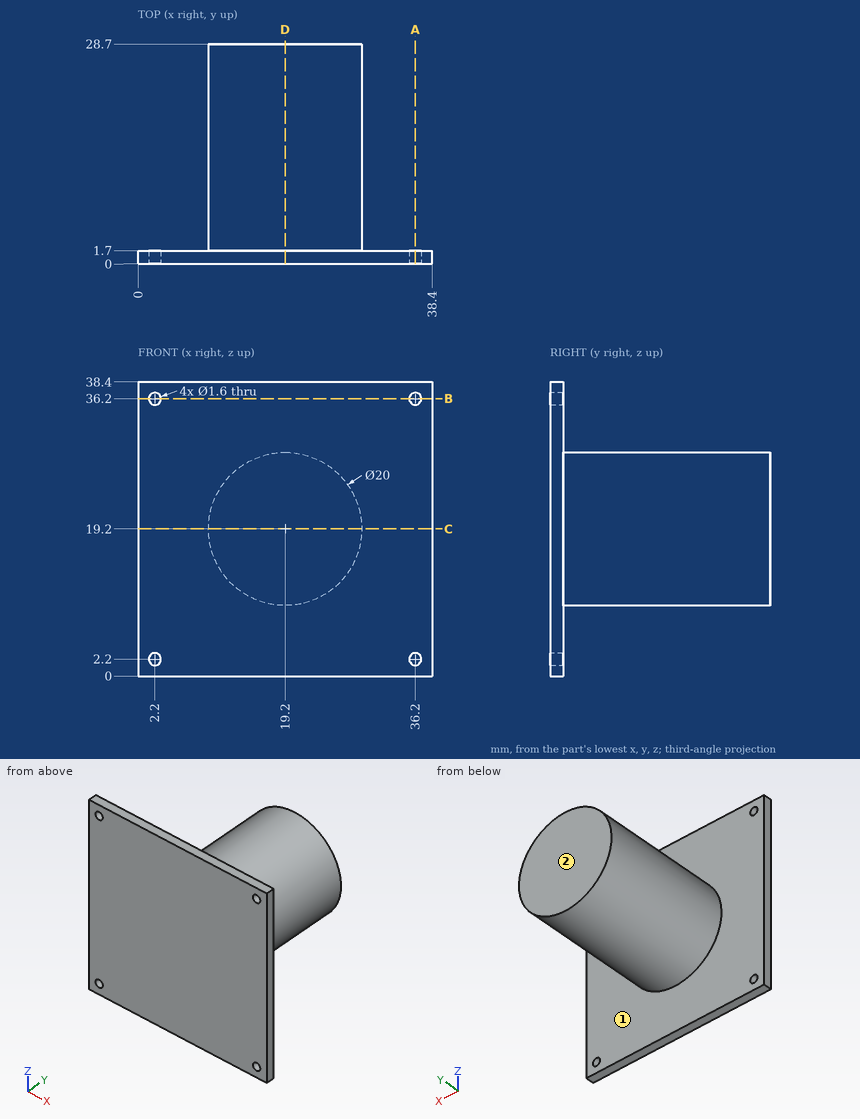
Geometry: see drawing. Coordinates: mm, zero at the bounding-box minimum. A direction names the side the tool comes from. Round coordinates to 2 decimals unless told otherwise and drop trailing zeros. Write each loop counter-clockwise with the first axis right and the second up, starting at its lowest first coordinate (ties: lowest second). Pieces come first, ordered by that corner, then holes.
Item 1: Material intervals for L1, parallel to X at y = 0.55, z = 2.2; L2, parallel to Y at x = 27, z = 4.5, sorted ascending.
Item 2: Section query A-A (x = 36.2). Return loops of the section in (y, z).
Item 3: Pin query (flat end, axial travel): P1, Ø1, axis at x = 24.5, z = 31, coming from the +Y side; P2, Ø1, axis at y = 7.5, z = 8.5, coming from the -X side. Return the tip coordinate at first contact, or that it passes through.
Item 4: Section query C-C (z = 19.2). Return loops of the section in (x, y), plus the area to 3 significant figures.
Item 5: Set-up query: the marked faces 1 and 2. Return all of +Z, -Z, +X, -X, +Y, -Y with unobstructed straight access to the full face (end or side cutting, diameter ignored); none if empty.
Item 6: Section query B-B (z = 36.2). Return loops of the section in (x, y), plus the area to 3 significant figures.
Item 7: Section query D-D (x = 19.2). Return loops of the section in (y, z), plus the area to 3 significant figures.
Completed:
1. L1: x = 0 to 1.4, 3 to 35.4, 37 to 38.4
1. L2: y = 0 to 1.7
2. outline: (0, 0) - (1.7, 0) - (1.7, 1.4) - (0, 1.4) - close; (0, 3) - (1.7, 3) - (1.7, 35.4) - (0, 35.4) - close; (0, 37) - (1.7, 37) - (1.7, 38.4) - (0, 38.4) - close
3. P1: stops at y = 1.7
3. P2: passes through
4. outline: (0, 0) - (38.4, 0) - (38.4, 1.7) - (29.2, 1.7) - (29.2, 28.7) - (9.2, 28.7) - (9.2, 1.7) - (0, 1.7) - close
4. area: 605 mm2
5. face 1: +Y
5. face 2: +Z, -Z, +X, -X, +Y
6. outline: (0, 0) - (1.4, 0) - (1.4, 1.7) - (0, 1.7) - close; (3, 0) - (35.4, 0) - (35.4, 1.7) - (3, 1.7) - close; (37, 0) - (38.4, 0) - (38.4, 1.7) - (37, 1.7) - close
6. area: 59.8 mm2
7. outline: (0, 0) - (1.7, 0) - (1.7, 9.2) - (28.7, 9.2) - (28.7, 29.2) - (1.7, 29.2) - (1.7, 38.4) - (0, 38.4) - close
7. area: 605 mm2
